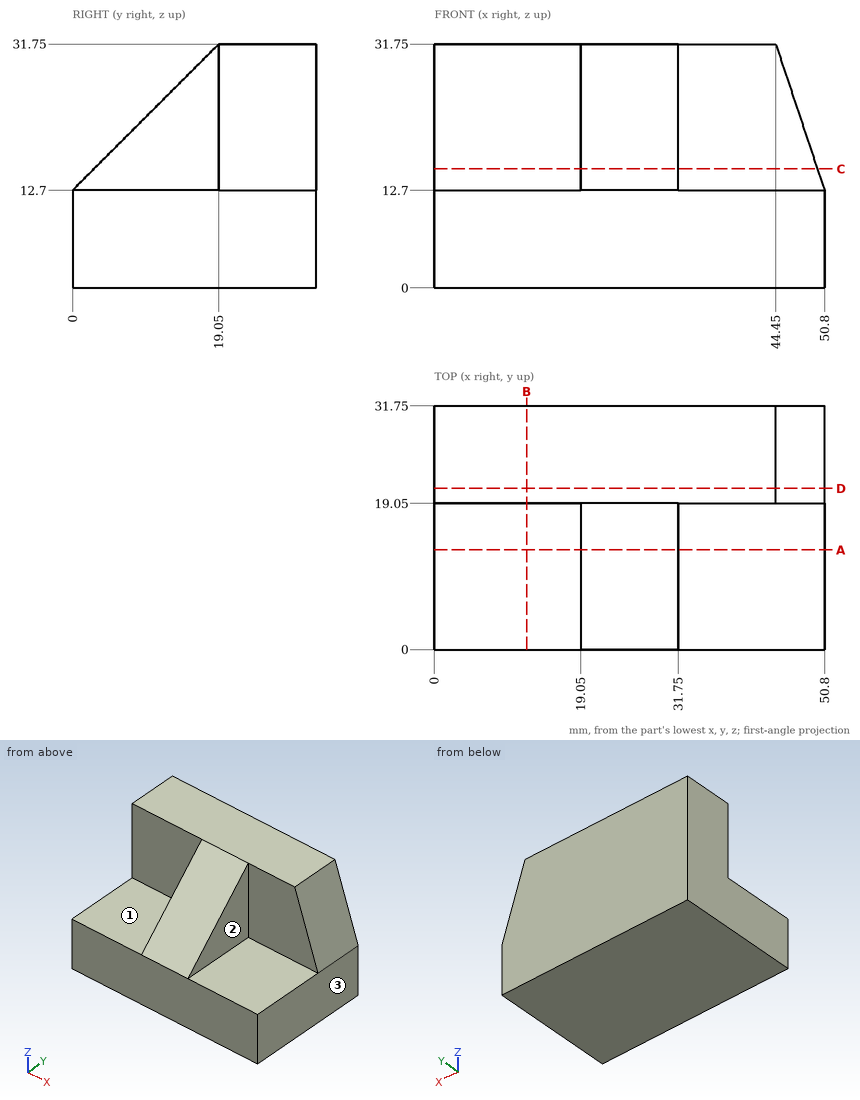
For this review, use the dimensioned drawing (mm, ordinates from the lowest corner) and the shaded views. A direction names the side the tool comes from. Round coordinates to 2 decimals unless told otherwise and drop trailing zeros. Write each loop counter-clockwise with the first axis right and the second up, starting at its lowest first coordinate (ties: lowest second). Pieces come first, ordered by that corner, then holes. Notation, with made-up numbers: M 27,78 L 70,78 A25 ccw 70,104 Z; hole C -38.5,69 d3. An arc over 180 degrees is marked long. Use CSV: the item, a comma, the result in double quotes. Start each with the question number.
(1) We need section D-D, the plane y = 21. State the section outline as (x, z) points, then the cut area to 3 significant figures.
(2) For line 1 along X through (y, z) = (10, 21); line 2 along Z through (x, y) = (13, 13), list the stretches that pass through material, from the lowest coordinate up.
(3) We need section A-A, the plane y = 13. State the section outline as (x, z) points.
(4) Tool access review of the marked faces 1, 2 and 3: name each direction out of +Z, -Z, +X, -X, +Y, -Y from which nothing blocks a thin tool from reaching the whole face with its end or side.
(5) We need section B-B, the plane x = 12. State the section outline as (y, z) points.
(6) We need section C-C, the plane z = 15.5. State the section outline as (x, y) points.
(7) Clearance check with flat-ended pins moving along their axes: P1, Ø5.5, axis at x = 10, y = 9, coming from the +Z side; P2, Ø15, axis at y = 8, z = 22, coming from the -X side; P3, Ø8, axis at y = 15, z = 15.5, coming from the -X side; P4, Ø9.5, axis at x = 41.5, z = 22, coming from the -Y side. State where each tip first meets the part, or that it passes through.
Findings:
1,outline,"M 0,0 L 50.8,0 L 50.8,12.7 L 44.45,31.75 L 0,31.75 Z"
1,area,"1,550 mm^2"
2,line 1,"19.05 to 31.75"
2,line 2,"0 to 12.7"
3,outline,"M 0,0 L 50.8,0 L 50.8,12.7 L 31.75,12.7 L 31.75,25.7 L 19.05,25.7 L 19.05,12.7 L 0,12.7 Z"
4,face 1,"+Z, -X, -Y"
4,face 2,"+Z, +X, -Y"
4,face 3,"+Z, -Z, +X, +Y, -Y"
5,outline,"M 0,0 L 31.75,0 L 31.75,31.75 L 19.05,31.75 L 19.05,12.7 L 0,12.7 Z"
6,outline,"M 0,19.05 L 19.05,19.05 L 19.05,2.8 L 31.75,2.8 L 31.75,19.05 L 49.87,19.05 L 49.87,31.75 L 0,31.75 Z"
7,P1,"z = 12.7"
7,P2,"x = 19.05"
7,P3,"x = 0"
7,P4,"y = 19.05"
